Design review of the part built by this model. Coordinates are the model's own, in mm. A direction names the side the tool comes from. Coordinates: 2 decimals unless noted, no trailing zeros. Write each loop counter-clockwise with the first axis right and the second up, starting at its lowest first coordinate (ties: lowest second). Pieces come first, ordered by that corner, then holes. Notation, with made-up numbers: (49, 4) -> (81, 4) arc R16 ccw to (81, 27) -> close; hole circle Ø9 at (54, 3.25). An arc over 180 degrees is marked (long way). Answer in a Markdown table with one row per item. Add a question column.
Item 1: Take a section at D-D, the plane x = 2.5. Write out the cut boundary in (y, z).
Item 2: Take a section at B-B, the plane y = 6.35. Write out the cut boundary in (x, z), and give its area (3 significant figures).
Item 3: Clearance check with flat-ended pins moving along their axes: P1, Ø1.5, axis at x = 0.5, z = 6.5, coming from the -Y side; P2, Ø1.5, axis at x = -1, y = 2, coming from the +Z side. State where each tip first meets the part, or that it passes through.
Item 4: Take a section at C-C, the plane z = 17. Write out the cut boundary in (x, y).
Item 5: For faces 1 (the face through (-1, 8, 16.51)), 2 (the face through (0, 12.7, 0)), list the 3-axis set-ups (+Z, -Z, +X, -X, +Y, -Y) from which the entire face can be reached by the end or side of a thin tool; tool diameter is ignored.
Item 6: To check wall thickness, follow line 1 (Z direction, x = -4.25, y = 11.25); line 2 (X direction, y = 0.5, z = 9.5); line 3 (Y direction, x = 4.75, z = -0.5). State the ranges of each line that lie inside material, in increasing order.
Autodesk Inventor part; units mm, degrees
ref_plane "YZ Plane" through (0, 0, 0) normal (1, 0, 0) x (0, 1, 0)
ref_plane "XZ Plane" through (0, 0, 0) normal (0, 1, 0) x (-1, 0, 0)
ref_plane "XY Plane" through (0, 0, 0) normal (0, 0, 1) x (1, 0, 0)
sketch "Sketch1" plane through (0, 0, 0) normal (0, 1, 0) x (-1, 0, 0)
  line L0 (-5.08, 16.51) -> (5.08, 16.51)
  line L1 (5.08, 16.51) -> (5.08, -16.51)
  line L2 (5.08, -16.51) -> (-5.08, -16.51)
  line L3 (-5.08, -16.51) -> (-5.08, 16.51)
  line L4 (-5.08, 16.51) -> (5.08, -16.51) construction
  line L5 (5.08, 16.51) -> (-5.08, -16.51) construction
  point P0 (0, 0)
  dimension "d0" = 10.16
  dimension "d1" = 33.02
extrude "Extrusion1" add sketch "Sketch1" along normal blind 12.7
fillet "Fillet1" radius 1.27 4 edges at (5.08, 12.7, 0) (5.08, 0, 0) (-5.08, 12.7, 0) (-5.08, 0, 0)
sketch "Sketch2" plane through (-3.81, 0, 16.51) normal (0, 0, 1) x (1, 0, 0)
  circle A0 centre (3.81, 6.35) radius 1.524
  point P0 (3.81, 0)
  dimension "d5" = 3.048
extrude "Extrusion2" add sketch "Sketch2" along normal blind 6.35
properties part number "mtr"
Answers:
| question | item | result |
|---|---|---|
| 1 | outline | (0, -16.51) -> (12.7, -16.51) -> (12.7, 16.51) -> (0, 16.51) -> close |
| 2 | outline | (-5.08, -16.51) -> (5.08, -16.51) -> (5.08, 16.51) -> (1.52, 16.51) -> (1.52, 22.86) -> (-1.52, 22.86) -> (-1.52, 16.51) -> (-5.08, 16.51) -> close |
| 2 | area | 355 mm^2 |
| 3 | P1 | stops at y = 0 |
| 3 | P2 | stops at z = 16.51 |
| 4 | outline | circle Ø3.05 at (0, 6.35) |
| 5 | face 1 | +Z |
| 5 | face 2 | +Z, -Z, +X, -X, +Y |
| 6 | line 1 | z = -16.51 to 16.51 |
| 6 | line 2 | x = -4.82 to 4.82 |
| 6 | line 3 | y = 0.42 to 12.28 |
